Design review of the part shown in the three views and the two pictorial views. Dimensions are in mm from the part's minimum x, y and z. Round coordinates to 2 decimals unless told otherwise and drop trailing zeros. Order: outer loops, then holes, each group sorted by start corner. A loop starts at its lowest first (then second) coordinate and runs counter-clockwise, first axis right, second up. Notation, with made-up numbers: (-23.75, 34) - (21.25, 34) arc R27 cw to (21.25, 64) - close; hole circle Ø5 at (3, 77). An arc over 180 degrees is marked (long way). One line per item, written item: value.
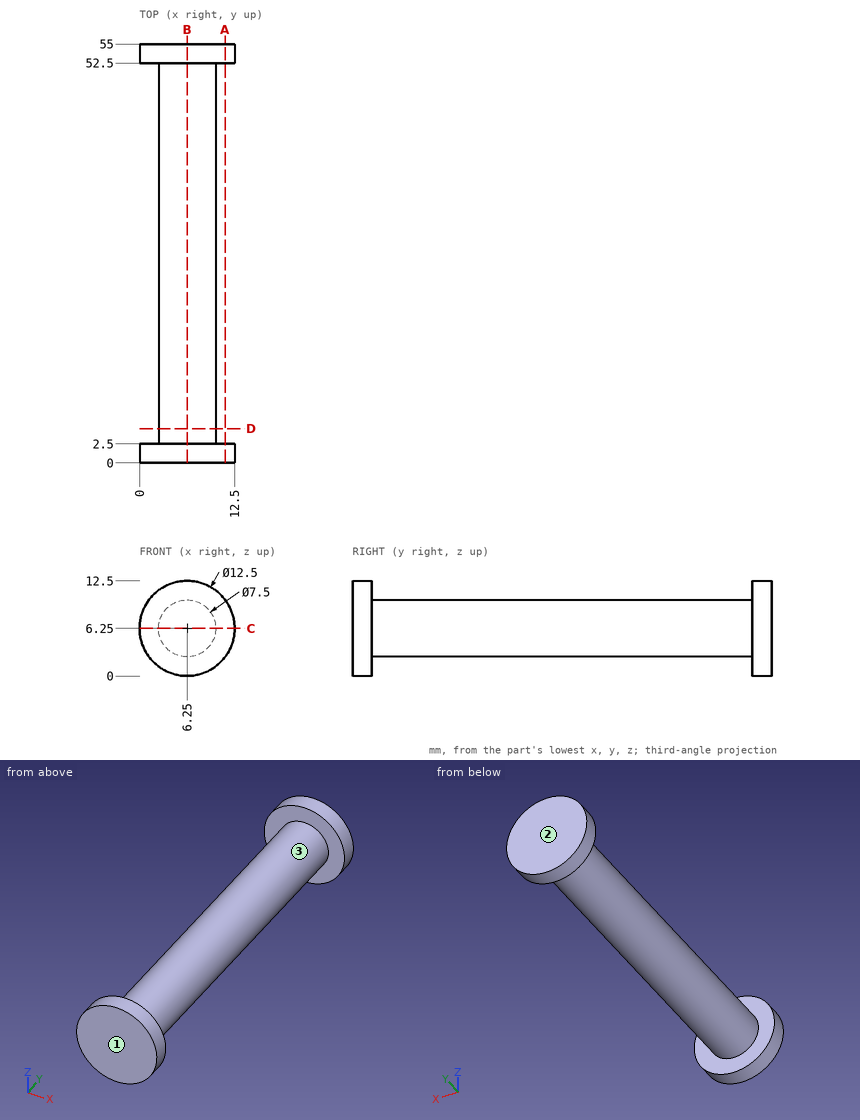
Item 1: Take a section at A-A (x = 11.25). Write out the cut boundary in (y, z).
Returned:
outline: (0, 2.5) - (2.5, 2.5) - (2.5, 10) - (0, 10) - close; (52.5, 2.5) - (55, 2.5) - (55, 10) - (52.5, 10) - close
Item 2: Wall thickness on line 1 (Y direction, x = 9.5, z = 2.75); line 2 (X direction, y = 9, z = 6); line 3 (Z direction, x = 5.25, y = 6): over which ranges is each line inside the solid? List them lowest first.
Returned:
line 1: 0 to 2.5, 52.5 to 55
line 2: 2.51 to 9.99
line 3: 2.64 to 9.86
Item 3: The part is to be moulded in two halves that separate along Y. For the marked faces 1, 2 and 3, say which applies: +Y half, -Y half, draft (parallel to the pull), parting line (faces both ways), or undercut.
Returned:
face 1: -Y half
face 2: +Y half
face 3: undercut
Item 4: Take a section at C-C (z = 6.25). Write out the cut boundary in (x, y), plus the area to 4 significant figures.
Returned:
outline: (0, 0) - (12.5, 0) - (12.5, 2.5) - (10, 2.5) - (10, 52.5) - (12.5, 52.5) - (12.5, 55) - (0, 55) - (0, 52.5) - (2.5, 52.5) - (2.5, 2.5) - (0, 2.5) - close
area: 437.5 mm^2
Item 5: Take a section at B-B (x = 6.25). Write out the cut boundary in (y, z), plus the area to 4 significant figures.
Returned:
outline: (0, 0) - (2.5, 0) - (2.5, 2.5) - (52.5, 2.5) - (52.5, 0) - (55, 0) - (55, 12.5) - (52.5, 12.5) - (52.5, 10) - (2.5, 10) - (2.5, 12.5) - (0, 12.5) - close
area: 437.5 mm^2
Item 6: Take a section at D-D (y = 4.5). Write out the cut boundary in (x, z), plus the area to 3 significant figures.
Returned:
outline: circle Ø7.5 at (6.25, 6.25)
area: 44.2 mm^2
Item 7: For P1, Ø3, axis at y = 41, z = 5, coming from the -X side; P2, Ø1, axis at y = 29, z = 4, coming from the +X side; P3, Ø1.5, axis at y = 36, z = 1.5, coming from the +X side, all flat-tipped, find the tip position at first contact; note any pin that passes through.
Returned:
P1: x = 2.5
P2: x = 9.57
P3: through
